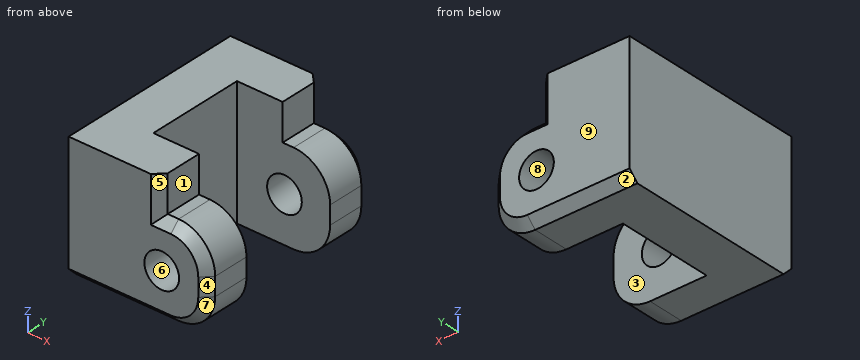
from build123d import *

# Parameters (mm, degrees)
SKETCH_1_R               = 6.25
EXTRUDE_1_DEPTH          = 15
SKETCH_2_W               = 29.5
SKETCH_2_H               = 20.7
EXTRUDE_2_DEPTH          = 5
SKETCH_3_W               = 39
SKETCH_3_H               = 20.7
SKETCH_3_R               = 1.6
EXTRUDE_3_DEPTH          = 5
SKETCH_4_W               = 10
SKETCH_4_H               = 5
EXTRUDE_4_DEPTH          = 10.2
SKETCH_5_R               = 1.9
CUT_EXTRUDE_1_DEPTH      = 21.7
FILLET_1_R               = 4
SKETCH_8_W               = 24
SKETCH_8_H               = 5
EXTRUDE_6_DEPTH          = 5
SKETCH_9_R               = 1.6
EXTRUDE_7_DEPTH          = 5
EXTRUDE_5_DEPTH          = 3
CHAMFER_1_SIZE           = 1
CHAMFER_2_SIZE           = 1
SKETCH_10_W              = 6.3
SKETCH_10_H              = 5.8
CUT_EXTRUDE_2_DEPTH      = 2.5
SKETCH_11_R              = 1.65
CUT_EXTRUDE_3_DEPTH      = 25.95
CUT_EXTRUDE_3_DEPTH_BACK = 15.75
CUT_EXTRUDE_4_DEPTH      = 1
CUT_EXTRUDE_4_DEPTH_BACK = 21.7


with BuildPart() as part:
    # ｽｹｯﾁ1 → ﾎﾞｽ - 押し出し1 (new body)
    with BuildSketch(Plane.XY):
        Circle(SKETCH_1_R)
    extrude(amount=-EXTRUDE_1_DEPTH)

    # ｽｹｯﾁ2 → ﾎﾞｽ - 押し出し2 (add)
    with BuildSketch(Plane.XY):
        Rectangle(SKETCH_2_W, SKETCH_2_H)
    extrude(amount=EXTRUDE_2_DEPTH)

    # ｽｹｯﾁ3 → ﾎﾞｽ - 押し出し3 (add)
    with BuildSketch(Plane(origin=(14.75, 0, 0), x_dir=(0, 0, -1), z_dir=(1, 0, 0))):
        with Locations((-24.5, 0)):
            Rectangle(SKETCH_3_W, SKETCH_3_H)
        with Locations((-20, 0)):
            Circle(SKETCH_3_R, mode=Mode.SUBTRACT)
    extrude(amount=-EXTRUDE_3_DEPTH)

    # ｽｹｯﾁ4 → ﾎﾞｽ - 押し出し4 (add)
    with BuildSketch(Plane(origin=(14.75, 0, 0), x_dir=(0, 0, -1), z_dir=(1, 0, 0))):
        with Locations((-5, 7.85)):
            Rectangle(SKETCH_4_W, SKETCH_4_H)
        with Locations((-5, -7.85)):
            Rectangle(SKETCH_4_W, SKETCH_4_H)
        with Locations((-39, 7.85)):
            Rectangle(SKETCH_4_W, SKETCH_4_H)
        with Locations((-39, -7.85)):
            Rectangle(SKETCH_4_W, SKETCH_4_H)
    extrude(amount=EXTRUDE_4_DEPTH)

    # ｽｹｯﾁ5 → ｶｯﾄ - 押し出し1 (cut, through all)
    with BuildSketch(Plane.XZ.offset(10.35)):
        with Locations((19.95, 5)):
            Circle(SKETCH_5_R)
        with Locations((19.95, 39)):
            Circle(SKETCH_5_R)
    extrude(amount=-CUT_EXTRUDE_1_DEPTH, mode=Mode.SUBTRACT)

    # ﾌｨﾚｯﾄ1
    fillet_1_edges = [part.edges().sort_by_distance(p)[0] for p in [
        (24.95, 7.85, 0),
        (24.95, 7.85, 10),
        (24.95, -7.85, 0),
        (24.95, -7.85, 10),
        (24.95, -7.85, 44),
        (24.95, -7.85, 34),
        (24.95, 7.85, 44),
        (24.95, 7.85, 34),
    ]]
    fillet(fillet_1_edges, radius=FILLET_1_R)

    # ｽｹｯﾁ8 → ﾎﾞｽ - 押し出し6 (add)
    with BuildSketch(Plane(origin=(14.75, 0, 0), x_dir=(0, 0, -1), z_dir=(1, 0, 0))):
        with Locations((-22, 7.85)):
            Rectangle(SKETCH_8_W, SKETCH_8_H)
        with Locations((-22, -7.85)):
            Rectangle(SKETCH_8_W, SKETCH_8_H)
    extrude(amount=EXTRUDE_6_DEPTH)

    # ｽｹｯﾁ9 → ﾎﾞｽ - 押し出し7 (add)
    with BuildSketch(Plane.ZY.offset(14.75)):
        with BuildLine():
            Line((5, 10.35), (11, 10.35))
            Line((11, 10.35), (22.121751649, 3.390895153))
            ThreePointArc((22.121751649, 3.390895153), (24, 0), (22.121751649, -3.390895153))
            Line((22.121751649, -3.390895153), (11, -10.35))
            Line((11, -10.35), (5, -10.35))
            Line((5, -10.35), (5, 10.35))
        make_face()
        with Locations((20, 0)):
            Circle(SKETCH_9_R, mode=Mode.SUBTRACT)
    extrude(amount=-EXTRUDE_7_DEPTH)

    # ｽｹｯﾁ6 → ﾎﾞｽ - 押し出し5 (add)
    with BuildSketch(Plane.XZ.offset(10.35)):
        Polygon((-9.75, 5), (9.75, 5), (9.75, 15), (-2.374355653, 8), (-9.75, 8), align=None)
    extrude_5 = extrude(amount=-EXTRUDE_5_DEPTH)

    # ﾐﾗｰ1: ﾎﾞｽ - 押し出し5 across plane
    add(extrude_5.mirror(Plane.ZX))

    # 面取り1
    chamfer_1_edges = [part.edges().sort_by_distance(p)[0] for p in [
        (20.35, -10.35, 34),
        (24.95, -10.35, 5),
        (20.35, -10.35, 10),
        (23.778427125, -10.35, 8.828427125),
        (23.778427125, -10.35, 1.171572875),
        (23.778427125, -10.35, 42.828427125),
        (23.778427125, -10.35, 35.171572875),
        (24.95, 10.35, 39),
        (3.1, 10.35, 0),
        (20.35, 10.35, 34),
        (20.35, 10.35, 10),
        (24.95, 10.35, 5),
        (23.778427125, 10.35, 1.171572875),
        (23.778427125, 10.35, 8.828427125),
        (23.778427125, 10.35, 42.828427125),
        (23.778427125, 10.35, 35.171572875),
        (19.75, 10.35, 22),
        (19.75, -10.35, 22),
        (9.75, -10.35, 29.5),
        (9.75, 0, 44),
        (15.35, -10.35, 44),
        (15.35, 10.35, 44),
        (9.75, 10.35, 29.5),
        (-14.75, 0, 0),
        (-14.75, 10.35, 5.5),
        (3.1, -10.35, 0),
        (-14.75, -10.35, 5.5),
        (24.95, -10.35, 39),
    ]]
    chamfer(chamfer_1_edges, length=CHAMFER_1_SIZE)

    # 面取り2
    chamfer_2_edges = [part.edges().sort_by_distance(p)[0] for p in [
        (-9.75, -8.85, 8),
        (-9.75, 8.85, 8),
    ]]
    chamfer(chamfer_2_edges, length=CHAMFER_2_SIZE)

    # ｽｹｯﾁ10 → ｶｯﾄ - 押し出し2 (cut)
    with BuildSketch(Plane(origin=(14.75, 0, 0), x_dir=(0, 0, -1), z_dir=(1, 0, 0))):
        with Locations((-20, 0)):
            Rectangle(SKETCH_10_W, SKETCH_10_H)
    extrude(amount=-CUT_EXTRUDE_2_DEPTH, mode=Mode.SUBTRACT)

    # ｽｹｯﾁ11 → ｶｯﾄ - 押し出し3 (cut, two sides)
    with BuildSketch(Plane(origin=(0, 0, 0), x_dir=(0, 0, -1), z_dir=(1, 0, 0))) as cut_extrude_3_sk:
        with Locations((7.5, 0)):
            Circle(SKETCH_11_R)
    extrude(amount=CUT_EXTRUDE_3_DEPTH, mode=Mode.SUBTRACT)
    extrude(cut_extrude_3_sk.sketch, amount=-CUT_EXTRUDE_3_DEPTH_BACK, mode=Mode.SUBTRACT)

    # ｽｹｯﾁ12 → ｶｯﾄ - 押し出し4 (cut, two sides)
    with BuildSketch(Plane(origin=(0, 10.35, 0), x_dir=(1, 0, 0), z_dir=(0, 1, 0))) as cut_extrude_4_sk:
        Polygon((147.57222826, -14), (29.932862948, -14), (9.75, -14), (9.75, 2.815371833), (9.75, 120.454737145), (-154.547009772, -47.957179489), (-16.724781512, -182.411916634), align=None)
    extrude(amount=CUT_EXTRUDE_4_DEPTH, mode=Mode.SUBTRACT)
    extrude(cut_extrude_4_sk.sketch, amount=-CUT_EXTRUDE_4_DEPTH_BACK, mode=Mode.SUBTRACT)


solid = part.part
Part model, mm, in its own coordinate system. Face numbers are marked on the shaded views. A direction names the side the tool comes from. Give positions to 0.01 mm unless a question says otherwise; leave off trailing zeros. Order: outer loops, then holes, each group sorted by start corner. A loop starts at its lowest first (then second) coordinate and runs counter-clockwise, first axis right, second up. Notation, with made-up numbers: (-9, -25.5) - (40, -25.5) arc R16 cw to (40, 1.5) - close; hole circle Ø11 at (83.5, 8). An arc over 180 degrees is marked (long way). One line per question, with ' | ' between items.
1. Drill centre lines: probe 1 along Z at (x, y) = (19.95, -9.05); probe 2 along Y at (x, z) = (22.5, 8.5); probe 3 along X at (y, z) = (5.25, 0.5). Where is each one in solid material? Low to high.
Filled in:
probe 1: 0 to 3.1, 6.9 to 10 | probe 2: -10.35 to -5.35, 5.35 to 10.35 | probe 3: 9.75 to 14.75
2. Band-saw the part on D-D on z = 11.5. List the corners of the cut face in (x, y), then the cut area to 4 significant figures.
Filled in:
outline: (9.75, -10.35) - (18.75, -10.35) - (19.75, -9.35) - (19.75, -5.35) - (14.75, -5.35) - (14.75, 5.35) - (19.75, 5.35) - (19.75, 9.35) - (18.75, 10.35) - (9.75, 10.35) - close | area: 152.5 mm²
3. Band-saw the part on B-B on x = 17.75. List the corners of the cut face in (y, z), then the cut area to 3 significant figures.
Filled in:
outline: (-10.35, 1) - (-9.35, 0) - (-5.35, 0) - (-5.35, 14) - (-10.35, 14) - close; (5.35, 0) - (9.35, 0) - (10.35, 1) - (10.35, 14) - (5.35, 14) - close | area: 139 mm²
4. Band-saw the part on A-A on z = 5. List the corners of the cut face in (x, y).
Filled in:
outline: (9.75, -10.35) - (18.05, -10.35) - (18.05, -5.35) - (14.75, -5.35) - (14.75, 5.35) - (18.05, 5.35) - (18.05, 10.35) - (9.75, 10.35) - close; (21.85, -10.35) - (23.95, -10.35) - (24.95, -9.35) - (24.95, -5.35) - (21.85, -5.35) - close; (21.85, 5.35) - (24.95, 5.35) - (24.95, 9.35) - (23.95, 10.35) - (21.85, 10.35) - close
5. Band-saw the part on C-C on x = 20. List the corners of the cut face in (y, z), then the cut area to 3 significant figures.
Filled in:
outline: (-10.35, 1) - (-9.35, 0) - (-5.35, 0) - (-5.35, 3.1) - (-10.35, 3.1) - close; (-10.35, 6.9) - (-5.35, 6.9) - (-5.35, 10) - (-9.35, 10) - (-10.35, 9) - close; (5.35, 0) - (9.35, 0) - (10.35, 1) - (10.35, 3.1) - (5.35, 3.1) - close; (5.35, 6.9) - (10.35, 6.9) - (10.35, 9) - (9.35, 10) - (5.35, 10) - close | area: 60.0 mm²
6. Pull direction X, two halves, no side cores. Call the marked faces 6, 7, 8 and 9: +X half, -X half, draft (parallel to the pull), parting line (faces both ways), or undercut.
Filled in:
face 6: undercut | face 7: +X half | face 8: undercut | face 9: draft
7. Drop flat-ended pins along their axis: P1, Ø4, axis at y = -2, z = 8.5, coming from the +X side; P2, Ø2, axis at y = -8, z = 11.5, coming from the +X side; P3, Ø0.6, axis at x = 20.5, y = -8, coming from the +Z side. Give the stop position or say it passes through.
Filled in:
P1: x = 14.75 | P2: x = 19.75 | P3: z = 10
8. Which spindle directions (+Z, -Z, +X, -X, +Y, -Y) get a long thin tool onto all of the face, cutting with end or side? Do the marked faces 1, 2, 3, 4 and 5. Say none if no direction does.
Filled in:
face 1: +Z, +X, +Y, -Y | face 2: -Z, +X, -X, +Y | face 3: +Z, -Z, +X | face 4: +Z, -Z, +X, -Y | face 5: +Z, +X, -Y
